Verification items for the finished model (mm, model axes). Face numbers are marked on the shaded views. A direction names the side the tool comes from. Coordinates: 2 decimals unless noted, no trailing zeros. Order: outer loops, then holes, each group sorted by start corner. A loop starts at its lowest first (then second) coordinate and runs counter-clockwise, first axis right, second up. Notation, with made-up numbers: (68, 36) - (102, 36) arc R18 cw to (102, 66) - close; hole circle Ø3 at (-20.75, 58.25). An arc over 180 degrees is marked (long way). Answer as CSV lines item,"result". Start each with the question number.
1. Section check D-D (z = 91). Record the cut outline in (x, y), and give its area (3 significant figures).
2. Go/stop test with flat-tipped pins: pin 1 (7.5 mm diameter, centred on y = -6.5, z = 105.5, fed in from -X); pin 2 (1 mm diameter, centred on x = 107, y = -3, fed in from +Z); pin 3 (5 mm diameter, centred on y = -4, z = 42, fed in from +X). Record where each tip stops, or that it passes through.
3. Section check C-C (y = -7.5). Count the separate pieces of the cut face and the enclosed holes in it, and give its area (3 significant figures).
4. Mould release check, pull along Z, two halves, no side actions. Record for the marked faces 4, 5, 6 and 7: pulls with the +Z half, pulls with the -Z half, needs draft (parallel to the pull), parting line crosses it, or undercut.
5. Material ranges on L1, parallel to Y at x = 43, z = 20; L2, parallel to Z at x = 42.45, y = -7.5; L3, parallel to X at y = -1.25, z = 81, recorded low to high. Write a range as [from, to].
6. Section check B-B (x = 9). Record the cut outline in (y, z), and give its area (3 significant figures).
7. Set-up check for the marked faces 1, 2 and 3: record each of +Z, -Z, +X, -X, +Y, -Y from which the full face is reachable in a straight line by a thin tool's end or side.
8. Section check A-A (z = 20). Record the cut outline in (x, y), and give its area (3 significant figures).
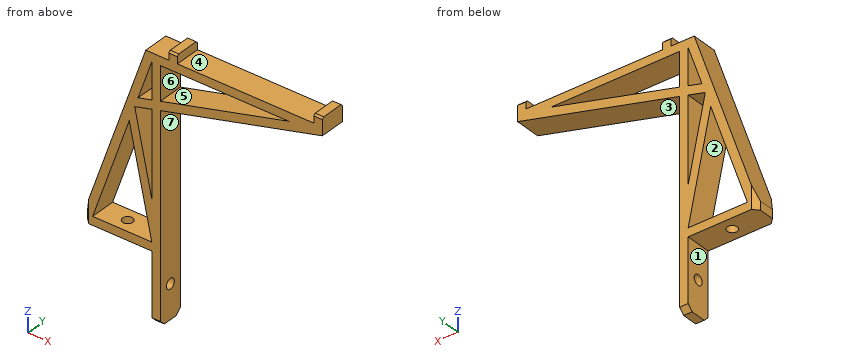
from build123d import *

# Parameters (mm, degrees)
PAD_DEPTH       = 15
SKETCH001_R     = 3
POCKET_DEPTH    = 5
SKETCH002_R     = 3
POCKET001_DEPTH = 5
CHAMFER_SIZE    = 1
CHAMFER001_SIZE = 3


with BuildPart() as part:
    # Sketch → Pad (new body)
    with BuildSketch(Plane.XZ):
        Polygon((40, 0), (40, 40), (0, 40), (0, 45), (36.44278, 150), (50, 150), (50, 155), (55, 155), (55, 150), (135, 150), (135, 155), (140, 155), (140, 145), (45, 120), (45, 0), align=None)
        Polygon((45, 145), (45, 125.170232), (120.353117, 145), align=None, mode=Mode.SUBTRACT)
        Polygon((40, 45), (26.782752, 106.918082), (5.29259, 45), align=None, mode=Mode.SUBTRACT)
        Polygon((40, 68.950927), (29.948406, 116.039054), (40, 118.684211), align=None, mode=Mode.SUBTRACT)
        Polygon((40, 123.854443), (31.923231, 121.728977), (40, 145), align=None, mode=Mode.SUBTRACT)
    extrude(amount=PAD_DEPTH)

    # Sketch001 (on Face2 of Pad) → Pocket (cut)
    with BuildSketch(Plane(origin=(0, 0, 40), x_dir=(1, 0, 0), z_dir=(0, 0, -1))):
        with Locations((20, 7.5)):
            Circle(SKETCH001_R)
    extrude(amount=-POCKET_DEPTH, mode=Mode.SUBTRACT)

    # Sketch002 (on Face1 of Pocket) → Pocket001 (cut)
    with BuildSketch(Plane(origin=(40, 0, 0), x_dir=(0, 0, -1), z_dir=(-1, 0, 0))):
        with Locations((-20, 7.5)):
            Circle(SKETCH002_R)
    extrude(amount=-POCKET001_DEPTH, mode=Mode.SUBTRACT)

    # Chamfer
    chamfer_edges = [part.edges().sort_by_distance(p)[0] for p in [
        (137.5, -15, 155),
        (137.5, 0, 155),
        (52.5, -15, 155),
        (52.5, 0, 155),
    ]]
    chamfer(chamfer_edges, length=CHAMFER_SIZE)

    # Chamfer001
    chamfer001_edges = [part.edges().sort_by_distance(p)[0] for p in [
        (42.5, -15, 0),
        (42.5, 0, 0),
        (0, -15, 42.5),
        (0, 0, 42.5),
    ]]
    chamfer(chamfer001_edges, length=CHAMFER001_SIZE)


solid = part.part
Evaluation:
1,outline,"(15.97, -15) - (21.26, -15) - (21.26, 0) - (15.97, 0) - close; (30.18, -15) - (35.29, -15) - (35.29, 0) - (30.18, 0) - close; (40, -15) - (45, -15) - (45, 0) - (40, 0) - close"
1,area,"231 mm²"
2,pin 1,"stops at x = 19.7"
2,pin 2,"stops at z = 150"
2,pin 3,"stops at x = 45"
3,separate pieces,"2"
3,enclosed holes,"3"
3,area,"2,730 mm²"
4,face 4,"pulls with the +Z half"
4,face 5,"undercut"
4,face 6,"undercut"
4,face 7,"needs draft"
5,L1,"y = [-15, -10.5], [-4.5, 0]"
5,L2,"z = [0, 17], [23, 150]"
5,L3,"x = [12.49, 17.79], [32.32, 37.43], [40, 45]"
6,outline,"(-15, 40) - (0, 40) - (0, 45) - (-15, 45) - close; (-15, 55.68) - (0, 55.68) - (0, 70.93) - (-15, 70.93) - close"
6,area,"304 mm²"
7,face 1,"-Z, -X, +Y, -Y"
7,face 2,"+Y, -Y"
7,face 3,"-Z, +X, +Y, -Y"
8,outline,"(40, -15) - (45, -15) - (45, -10.5) - (40, -10.5) - close; (40, -4.5) - (45, -4.5) - (45, 0) - (40, 0) - close"
8,area,"45.0 mm²"
